Here's how the part is built. I have some questions about the finished solid (model axes, mm). A direction names the side the tool comes from. Round coordinates to 2 decimals unless told otherwise and drop trailing zeros. Write each loop counter-clockwise with the first axis right and the second up, starting at its lowest first coordinate (ties: lowest second). Pieces come first, ordered by that corner, then holes. Notation, with made-up numbers: M 47,19.5 L 89,19.5 A22 cw 89,25.5 Z; hole C 31,-20 d1. An arc over 180 degrees is marked long. Write item = value, one per line. Start each with the question number.
(1) I want a section at D-D (y = 9). List the corners of the cut face in (x, z) for me, and give its area (3 significant figures).
(2) I want a section at C-C (x = -9.5). List the corners of the cut face in (y, z) for me.
(3) I want a section at A-A (x = 0). List the corners of the cut face in (y, z) for me.
(4) Will these pins go through, and if not, where does the flat tip stop? pin 1 Ø8 at (x, y) = (14, 7) entering from +Z; pin 2 Ø6 at (x, y) = (-13.5, 2.5) entering from +Z; pin 3 Ø5 at (x, z) = (10.39, 6) entering from -Y.
(5) I want a section at B-B (y = 2). List the corners of the cut face in (x, z) for me, and give its area (3 significant figures).
(6) On a 3-axis mill with a long thin cutter (end or side, diameter ignored), from which of +Z, -Z, +X, -X, +Y, -Y can I reach the whole of each face in a straight line? I mean faces 1 (the flat face through (4, 4, -4)), 2 (the cylindrical face through (0, 5, -2)), 3 (the cylindrical face through (-14.985, 12.028, -0.66)). Say none if no direction works.
(7) If we mould it in two halves opening along Z, with no side actions, what happens to faces 4 (the cylindrical face through (-1.08, 1.97, -4.88)), 5 (the cylindrical face through (20.03, 6.9, -6.31)), 6 (the cylindrical face through (8.767, 1.972, -16.856)), 7 (the flat face through (9, 14, 14))? For each: released by +Z, released by -Z, zero draft, split by the parting line, or undercut.
(8) I need wall thicknesses on line 1 along Z through (x, y) = (0, 6); line 2 along Z through (x, y) = (0, 3.2); line 3 along X through (y, z) = (12.6, 0). Which ranges of each line are inside material? Lowest first, please.
```python
from build123d import *

# Parameters (mm, degrees)
SKETCH1_R           = 21
BOSS_EXTRUDE1_DEPTH = 14
SKETCH2_R           = 15
CUT_EXTRUDE1_DEPTH  = 4
SKETCH3_R           = 19
SKETCH3_R_2         = 5
CUT_EXTRUDE2_DEPTH  = 4
SKETCH4_R           = 2
CUT_EXTRUDE3_DEPTH  = 15
SKETCH5_R           = 2
CUT_EXTRUDE4_DEPTH  = 11


with BuildPart() as part:
    # Sketch1 → Boss-Extrude1 (new body)
    with BuildSketch(Plane(origin=(0, 0, 0), x_dir=(1, 0, 0), z_dir=(0, 1, 0))):
        Circle(SKETCH1_R)
    extrude(amount=BOSS_EXTRUDE1_DEPTH)

    # Sketch2 → Cut-Extrude1 (cut)
    with BuildSketch(Plane(origin=(0, 14, 0), x_dir=(1, 0, 0), z_dir=(0, 1, 0))):
        Circle(SKETCH2_R)
    extrude(amount=-CUT_EXTRUDE1_DEPTH, mode=Mode.SUBTRACT)

    # Sketch3 → Cut-Extrude2 (cut)
    with BuildSketch(Plane.XZ):
        Circle(SKETCH3_R)
        Circle(SKETCH3_R_2, mode=Mode.SUBTRACT)
    extrude(amount=-CUT_EXTRUDE2_DEPTH, mode=Mode.SUBTRACT)

    # Sketch4 → Cut-Extrude3 (cut, through all)
    with BuildSketch(Plane.XZ):
        Circle(SKETCH4_R)
    extrude(amount=-CUT_EXTRUDE3_DEPTH, mode=Mode.SUBTRACT)

    # Sketch5 → Cut-Extrude4 (cut, through all)
    with BuildSketch(Plane.XZ.offset(-4)):
        with Locations((0, 12)):
            Circle(SKETCH5_R)
        with Locations((10.392304845, 6)):
            Circle(SKETCH5_R)
        with Locations((10.392304845, -6)):
            Circle(SKETCH5_R)
        with Locations((0, -12)):
            Circle(SKETCH5_R)
        with Locations((-10.392304845, -6)):
            Circle(SKETCH5_R)
        with Locations((-10.392304845, 6)):
            Circle(SKETCH5_R)
    extrude(amount=-CUT_EXTRUDE4_DEPTH, mode=Mode.SUBTRACT)


solid = part.part
```
Returned:
q1.outline = C 0,0 d42; hole C -10.39,-6 d4; hole C -10.39,6 d4; hole C 0,-12 d4; hole C 0,0 d4; hole C 0,12 d4; hole C 10.39,-6 d4; hole C 10.39,6 d4
q1.area = 1,300 mm²
q2.outline = M 0,-18.73 L 14,-18.73 L 14,-11.61 L 10,-11.61 L 10,-7.79 L 4,-7.79 L 4,-16.45 L 0,-16.45 Z; M 0,16.45 L 4,16.45 L 4,7.79 L 10,7.79 L 10,11.61 L 14,11.61 L 14,18.73 L 0,18.73 Z; M 4,-4.21 L 10,-4.21 L 10,4.21 L 4,4.21 Z
q3.outline = M 0,-21 L 14,-21 L 14,-15 L 10,-15 L 10,-14 L 4,-14 L 4,-19 L 0,-19 Z; M 0,-5 L 4,-5 L 4,-10 L 10,-10 L 10,-2 L 0,-2 Z; M 0,2 L 10,2 L 10,10 L 4,10 L 4,5 L 0,5 Z; M 0,19 L 4,19 L 4,14 L 10,14 L 10,15 L 14,15 L 14,21 L 0,21 Z
q4.pin_1 = 18.47
q4.pin_2 = 18.19
q4.pin_3 = 4
q5.outline = C 0,0 d42; C 0,0 d10; hole C 0,0 d38; hole C 0,0 d4
q5.area = 317 mm²
q6.face_1 = -Y
q6.face_2 = +Y, -Y
q6.face_3 = +Y
q7.face_4 = undercut
q7.face_5 = split by the parting line
q7.face_6 = undercut
q7.face_7 = zero draft
q8.line_1 = -21 to -14, -10 to -2, 2 to 10, 14 to 21
q8.line_2 = -21 to -19, -5 to -2, 2 to 5, 19 to 21
q8.line_3 = -21 to -15, 15 to 21
